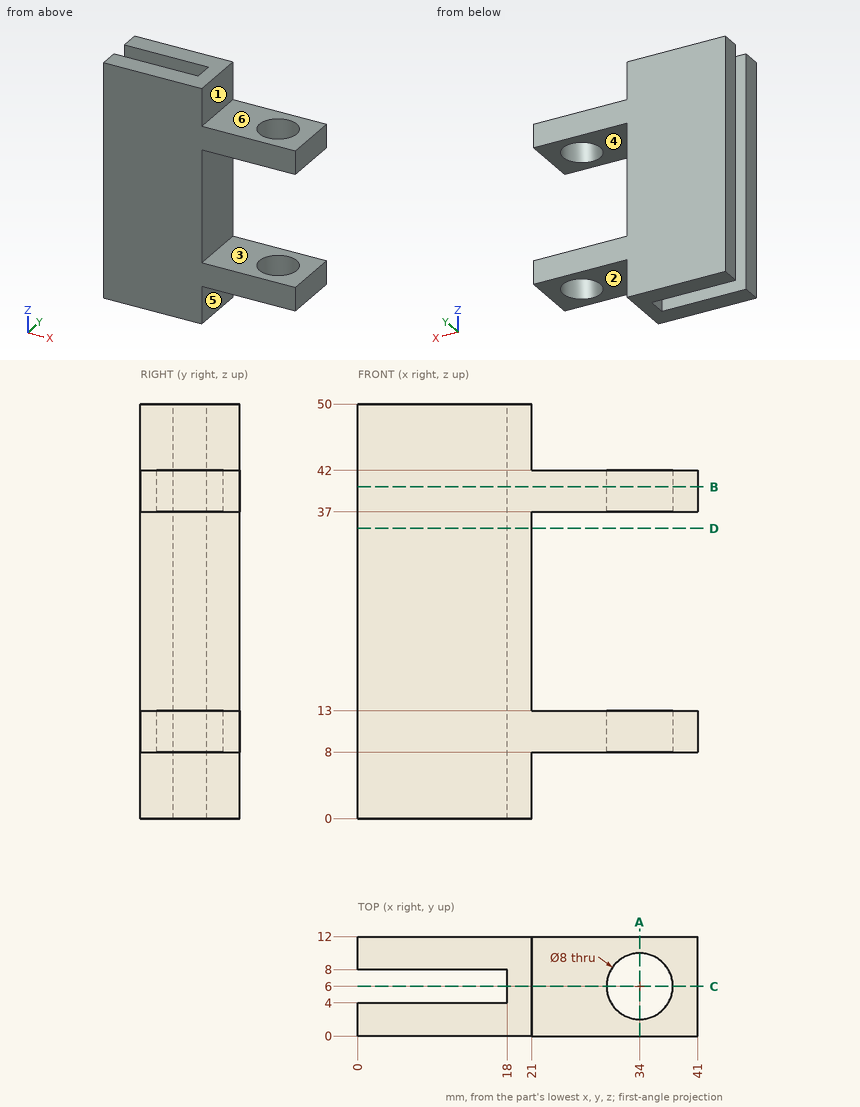
The figure shows three views and two pictorial views of one solid part (mm, origin at its lowest corner). Answer the questions. A direction names the side the tool comes from. Coordinates: 2 decimals unless noted, no trailing zeros. Loops run counter-clockwise (first coordinate to the right, second up) from the corner with the lowest first, then second, coordinate; pieces in that order, holes last. Notation, with made-up numbers: (37, 14) -> (77, 14) arc R13 cw to (77, 24) -> close; hole circle Ø8 at (47.5, 77). An arc over 180 degrees is marked (long way). Return JSON: item names as keys, results as strings. Group by question number.
(1) Find the intervals of material crossed by probe 1 along Z at (x, y) = (21.5, 6.5); probe 2 along Y at (x, z) = (34, 10); probe 3 along X at (y, z) = (7.75, 18), in increasing order. Write a range as from..to.
(2) A cutting plane is placed at D-D on z = 35. Write down the section's boundary in (x, y).
(3) A cutting plane is placed at B-B on z = 40. Write down the section's boundary in (x, y), and give its area (3 significant figures).
(4) Which of the six approach directions +Z, -Z, +X, -X, +Y, -Y give full straight-line access (tool end or side, diameter ignored) to the marked faces 4, 5 and 6?
(5) Given pin 1 Ø3.5 at (x, y) = (31, 6.5) entering from -Z; pin 2 Ø2 at (y, z) = (7.5, 44.5) entering from +X; pin 3 Ø6 at (x, y) = (31, 3) entering from +Z; pin 4 Ø1 at (x, y) = (15.5, 7) entering from -Z, each flat-ended and moving along its own axis, determine where each tip first touches the part or whether it passes through.
(6) A cutting plane is placed at C-C on y = 6. Write down the section's boundary in (x, z), and give its area (3 significant figures).
(7) Determine the mould class of the marked faces 1, 2 and 3 for opening direction Z: released by +Z, released by -Z, zero draft, split by the parting line, or undercut.
(8) A cutting plane is placed at A-A on x = 34. Write down the section's boundary in (y, z), and give its area (3 significant figures).
The answers:
{
 "1": {"probe 1": "z = 8..13, 37..42", "probe 2": "y = 0..2, 10..12", "probe 3": "x = 18..21"},
 "2": {"outline": "(0, 0) -> (21, 0) -> (21, 12) -> (0, 12) -> (0, 8) -> (18, 8) -> (18, 4) -> (0, 4) -> close"},
 "3": {"outline": "(0, 0) -> (41, 0) -> (41, 12) -> (0, 12) -> (0, 8) -> (18, 8) -> (18, 4) -> (0, 4) -> close; hole circle Ø8 at (34, 6)", "area": "370 mm^2"},
 "4": {"face 4": "+X, +Y, -Y", "face 5": "-Z, +X, +Y, -Y", "face 6": "+Z, +X, +Y, -Y"},
 "5": {"pin 1": "stops at z = 8", "pin 2": "stops at x = 21", "pin 3": "stops at z = 42", "pin 4": "passes through"},
 "6": {"outline": "(18, 0) -> (21, 0) -> (21, 8) -> (30, 8) -> (30, 13) -> (21, 13) -> (21, 37) -> (30, 37) -> (30, 42) -> (21, 42) -> (21, 50) -> (18, 50) -> close; (38, 8) -> (41, 8) -> (41, 13) -> (38, 13) -> close; (38, 37) -> (41, 37) -> (41, 42) -> (38, 42) -> close", "area": "270 mm^2"},
 "7": {"face 1": "zero draft", "face 2": "released by -Z", "face 3": "undercut"},
 "8": {"outline": "(0, 8) -> (2, 8) -> (2, 13) -> (0, 13) -> close; (0, 37) -> (2, 37) -> (2, 42) -> (0, 42) -> close; (10, 8) -> (12, 8) -> (12, 13) -> (10, 13) -> close; (10, 37) -> (12, 37) -> (12, 42) -> (10, 42) -> close", "area": "40.0 mm^2"}
}
